```python
from build123d import *

# Parameters (mm, degrees)
SKETCH_1_W          = 170
SKETCH_1_H          = 55.5
EXTRUDE_1_DEPTH     = 3
SKETCH_2_R          = 1.5
CUT_EXTRUDE_1_DEPTH = 3
CUT_EXTRUDE_2_DEPTH = 3
FILLET_1_R          = 5
SKETCH_4_R          = 1.5
CUT_EXTRUDE_3_DEPTH = 3
CHAMFER_1_SIZE      = 0.5


with BuildPart() as part:
    # 草图1 → 凸台-拉伸1 (new body)
    with BuildSketch(Plane.XY):
        with Locations((-15, -12.75)):
            Rectangle(SKETCH_1_W, SKETCH_1_H)
    extrude(amount=EXTRUDE_1_DEPTH)

    # 草图2 → 切除-拉伸1 (cut)
    with BuildSketch(Plane.XY.offset(3)):
        with Locations((60, -15.5)):
            Circle(SKETCH_2_R)
        with Locations((-60, -15.5)):
            Circle(SKETCH_2_R)
    extrude(amount=-CUT_EXTRUDE_1_DEPTH, mode=Mode.SUBTRACT)

    # 草图3 → 切除-拉伸2 (cut)
    with BuildSketch(Plane.XY.offset(3)):
        with BuildLine():
            Line((-20, -15.5), (5, -15.5))
            ThreePointArc((5, -15.5), (15.606601718, -11.106601718), (20, -0.5))
            Line((20, -0.5), (20, 15))
            Line((20, 15), (-35, 15))
            Line((-35, 15), (-35, -0.5))
            ThreePointArc((-35, -0.5), (-30.606601718, -11.106601718), (-20, -15.5))
        make_face()
    extrude(amount=-CUT_EXTRUDE_2_DEPTH, mode=Mode.SUBTRACT)

    # 圆角1
    fillet_1_edges = [part.edges().sort_by_distance(p)[0] for p in [
        (70, -40.5, 1.5),
        (-100, -40.5, 1.5),
    ]]
    fillet(fillet_1_edges, radius=FILLET_1_R)

    # 草图4 → 切除-拉伸3 (cut)
    with BuildSketch(Plane.XY.offset(3)):
        with Locations((-95, -15.5)):
            Circle(SKETCH_4_R)
    extrude(amount=-CUT_EXTRUDE_3_DEPTH, mode=Mode.SUBTRACT)

    # 倒角1
    chamfer_1_edges = [part.edges().sort_by_distance(p)[0] for p in [
        (45, 15, 3),
        (-67.5, 15, 0),
        (-67.5, 15, 3),
        (45, 15, 0),
    ]]
    chamfer(chamfer_1_edges, length=CHAMFER_1_SIZE)


solid = part.part
```
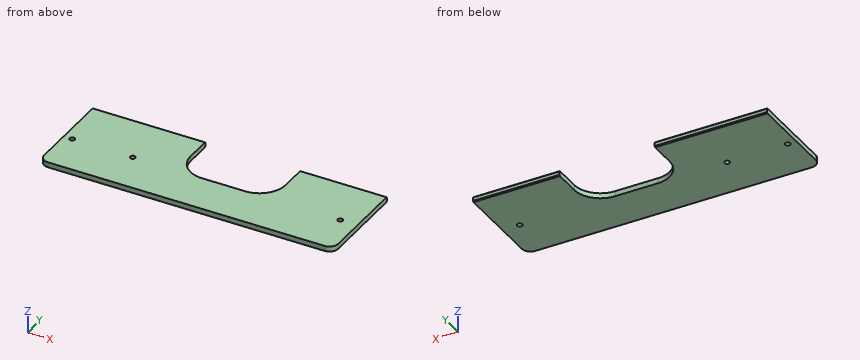
Read the model definition and answer for the solid it produces. Units are mm, in the model's axes. Round coordinates to 2 decimals unless told otherwise and drop trailing zeros. Write each loop counter-clockwise with the first axis right and the second up, starting at its lowest first coordinate (ties: lowest second). Pieces come first, ordered by that corner, then holes. Notation, with made-up numbers: (64.25, 3) - (69.25, 3) arc R30 cw to (69.25, 31) - close; hole circle Ø5 at (0.5, -22). An arc over 180 degrees is marked (long way). One line per item, written item: value.
Q1. Straight lines are drawn through the part: line 1 (X direction, y = 2.5, z = 1.9); line 2 (Y direction, x = -60, z = 1); line 3 (X direction, y = -16.5, z = 0.2). For each, find the intervals that lie inside material, in ascending order. Write a range as from..to.
The answers:
line 1: x = -100..-35, 20..70
line 2: y = -40.5..-17, -14..15
line 3: x = -100..-96.12, -93.88..-61.12, -58.88..58.88, 61.12..70
Q2. Find section B-B (y = 8). Determine the outline of the cut face in (x, z), and give its area (3 significant figures).
The answers:
outline: (-100, 0) - (-35, 0) - (-35, 3) - (-100, 3) - close; (20, 0) - (70, 0) - (70, 3) - (20, 3) - close
area: 345 mm2
Q3. Find section C-C (z = 1.35). Determine the outline of the cut face in (x, y), and give its area (3 significant figures).
The answers:
outline: (-100, -35.5) arc R5 ccw to (-95, -40.5) - (65, -40.5) arc R5 ccw to (70, -35.5) - (70, 15) - (20, 15) - (20, -0.5) arc R15 cw to (5, -15.5) - (-20, -15.5) arc R15 cw to (-35, -0.5) - (-35, 15) - (-100, 15) - close; hole circle Ø3 at (-95, -15.5); hole circle Ø3 at (-60, -15.5); hole circle Ø3 at (60, -15.5)
area: 7,820 mm2
Q4. Find section D-D (y = -6.5). Determine the outline of the cut face in (x, z).
The answers:
outline: (-100, 0) - (-33.75, 0) - (-33.75, 3) - (-100, 3) - close; (18.75, 0) - (70, 0) - (70, 3) - (18.75, 3) - close
Q5. Find section A-A (x = -60). Determine the outline of the cut face in (y, z), and give its area (3 significant figures).
The answers:
outline: (-40.5, 0) - (-17, 0) - (-17, 3) - (-40.5, 3) - close; (-14, 0) - (14.5, 0) - (15, 0.5) - (15, 2.5) - (14.5, 3) - (-14, 3) - close
area: 157 mm2
